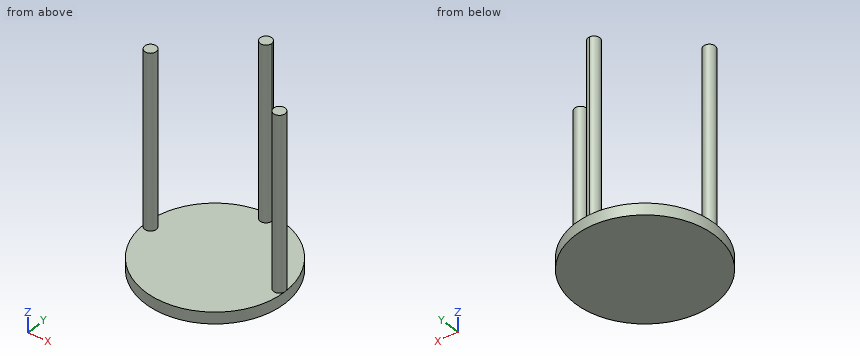
from build123d import *

# Parameters (mm, degrees)
F0_R     = 76.2
F1_DEPTH = 12.7
F2_R     = 6.35
F3_DEPTH = 190.5


with BuildPart() as f1:
    # F0 (on Top) → F1 (new body)
    with BuildSketch(Plane.XY):
        Circle(F0_R)
    extrude(amount=F1_DEPTH)

    # F2 (on face) → F3 (join)
    with BuildSketch(Plane.XY.offset(12.7)):
        with BuildLine():
            ThreePointArc((-63.5, 0), (-69.85, 6.35), (-76.2, 0))
            ThreePointArc((-76.2, 0), (-69.85, -6.35), (-63.5, 0))
        make_face()
        with BuildLine():
            ThreePointArc((0, 76.2), (-4.490128, 65.359872), (6.35, 69.85))
            ThreePointArc((6.35, 69.85), (4.490128, 74.340128), (0, 76.2))
        make_face()
        with Locations((69.85, 0)):
            Circle(F2_R)
    extrude(amount=F3_DEPTH)


solid = f1.part
CAD build for the part. Positions are in the model's coordinates, mm. Coordinates: 2 decimals unless noted, no trailing zeros. Order: outer loops, then holes, each group sorted by start corner. A loop starts at its lowest first (then second) coordinate and runs counter-clockwise, first axis right, second up.
Item 1: Band-saw the part on B-B on x = 69.85. List the corners of the cut face in (y, z), plus the area to 3 significant figures.
Check sheet entries:
outline: (-30.45, 0) - (30.45, 0) - (30.45, 12.7) - (6.35, 12.7) - (6.35, 203.2) - (-6.35, 203.2) - (-6.35, 12.7) - (-30.45, 12.7) - close
area: 3,190 mm2
Item 2: Band-saw the part on A-A on z = 176.5. List the corners of the cut face in (x, y).
Check sheet entries:
outline: circle Ø12.7 at (-69.85, 0); circle Ø12.7 at (0, 69.85); circle Ø12.7 at (69.85, 0)
Item 3: Pin check, flat tips, straight feed: pin 1 Ø12 at (y, z) = (54.5, 22) entering from -X; pin 2 Ø4 at (x, y) = (35, 14) entering from +Z. Stop position of each tip, or through.
Check sheet entries:
pin 1: passes through
pin 2: stops at z = 12.7
Item 4: Band-saw the part on C-C on y = -11.5. List the corners of the cut face in (x, z), plus the area to 3 significant figures.
Check sheet entries:
outline: (-75.33, 0) - (75.33, 0) - (75.33, 12.7) - (-75.33, 12.7) - close
area: 1,910 mm2
Item 5: Band-saw the part on D-D on y = 47. List the corners of the cut face in (x, z).
Check sheet entries:
outline: (-59.98, 0) - (59.98, 0) - (59.98, 12.7) - (-59.98, 12.7) - close
Item 6: Drill centre lines: L1, parallel to Z at x = -59.5, y = 5.5; L2, parallel to X at y = 70.5, z = 21; L3, parallel to X at y = -1, z = 125. Where is each one in solid material? Low to high.
Check sheet entries:
L1: z = 0 to 12.7
L2: x = -6.32 to 6.32
L3: x = -76.12 to -63.58, 63.58 to 76.12
